Geometry check sheet. Reference: the model listing, model coordinates, mm. A direction names the side the tool comes from. Give positions to 0.01 mm unless a question says otherwise; leave off trailing zeros. Order: outer loops, then holes, each group sorted by start corner. A loop starts at its lowest first (then second) coordinate and runs counter-clockwise, first axis right, second up. Notation, with made-up numbers: M 52,79.25 L 101,79.25 A20 ccw 101,96.25 Z; hole C 50,0 d7. An arc over 180 degrees is marked long. Put each result on its own line as item: value. Start each with the question number.
Q1. Section check A-A on z = 0. Record the cut outline in (x, y).
Q2. Section check C-C on y = 18. Record the cut outline in (x, z).
Q3. Go/stop test with flat-tipped pins: pin 1 (2 mm diameter, centred on x = -42.5, z = -20, fed in from -Y); pin 2 (10 mm diameter, centred on y = 42.5, z = -3.5, fed in from -X). Record where each tip stops, or that it passes through.
Q4. Mould release check, pull along Z, two halves, no side actions. Record for faces 3 (the cylindrical face through (64.06, 36.12, 49.43)), 4 (the flat face through (18, 6, -60)): +Z half, -Z half, draft (parallel to the pull), parting line (faces both ways), or undercut.
Q5. Section check D-D on x = -36. Record the cut outline in (y, z).
Q6. Material ranges on L1, parallel to X at y = 46, z = 29; L2, parallel to Y at x = -27.5, z = 23; L3, parallel to Y at x = -37.5, z = 51, recorded low to high.
Q7. Section check B-B on x = 0. Record the cut outline in (y, z).
Q8. Access from +Z, -Z, +X, -X, +Y, -Y to the whole of each face (thin tool, end or side, straight path). Record for faces 1 (the flat face through (-60, 4, 1)), 2 (the flat face through (60, 29, 1)).
```python
from build123d import *

# Parameters (mm, degrees)
SKETCH_1_W          = 120
SKETCH_1_H          = 120
EXTRUDE_1_DEPTH     = 8
SKETCH_2_W          = 120
SKETCH_2_H          = 50
EXTRUDE_2_DEPTH     = 8
SKETCH_3_R          = 12.5
CUT_EXTRUDE_1_DEPTH = 8
SKETCH_4_R          = 55
CUT_EXTRUDE_2_DEPTH = 0.1


with BuildPart() as part:
    # 草图1 → 凸台-拉伸1 (new body)
    with BuildSketch(Plane(origin=(0, 0, 0), x_dir=(1, 0, 0), z_dir=(0, 1, 0))):
        Rectangle(SKETCH_1_W, SKETCH_1_H)
    extrude(amount=EXTRUDE_1_DEPTH)

    # 草图2 → 凸台-拉伸2 (add)
    with BuildSketch(Plane(origin=(60, 0, 0), x_dir=(0, 0, -1), z_dir=(1, 0, 0))):
        with Locations((0, 25)):
            Rectangle(SKETCH_2_W, SKETCH_2_H)
    extrude(amount=EXTRUDE_2_DEPTH)

    # 草图3 → 切除-拉伸1 (cut)
    with BuildSketch(Plane(origin=(68, 0, 0), x_dir=(0, 0, -1), z_dir=(1, 0, 0))):
        with Locations((-40.221925454, 27.667787736)):
            Circle(SKETCH_3_R)
        with Locations((37.778074521, 27.665810834)):
            Circle(SKETCH_3_R)
    extrude(amount=-CUT_EXTRUDE_1_DEPTH, mode=Mode.SUBTRACT)

    # 草图4 → 切除-拉伸2 (cut)
    with BuildSketch(Plane.XZ):
        with Locations(Location((0, 0, 0), (0, 0, 270))):
            Circle(SKETCH_4_R)
    extrude(amount=-CUT_EXTRUDE_2_DEPTH, mode=Mode.SUBTRACT)


solid = part.part
```
Results found:
1. outline: M -60,0 L -55,0 L -55,0.1 L 55,0.1 L 55,0 L 68,0 L 68,50 L 60,50 L 60,8 L -60,8 Z
2. outline: M 60,-60 L 68,-60 L 68,-45.7 L 60,-45.7 Z; M 60,-29.85 L 68,-29.85 L 68,32.3 L 60,32.3 Z; M 60,48.15 L 68,48.15 L 68,60 L 60,60 Z
3. pin 1: stops at y = 0.1
3. pin 2: stops at x = 60
4. face 3: undercut
4. face 4: -Z half
5. outline: M 0,-60 L 8,-60 L 8,60 L 0,60 L 0,41.58 L 0.1,41.58 L 0.1,-41.58 L 0,-41.58 Z
6. L1: x = 60 to 68
6. L2: y = 0.1 to 8
6. L3: y = 0 to 8
7. outline: M 0,-60 L 8,-60 L 8,60 L 0,60 L 0,55 L 0.1,55 L 0.1,-55 L 0,-55 Z
8. face 1: +Z, -Z, -X, +Y, -Y
8. face 2: +Z, -Z, -X, +Y
